```python
from build123d import *

# Parameters (mm, degrees)
F1_DEPTH = 1
F3_DEPTH = 2
F4_W     = 19.942
F4_H     = 20.917
F5_DEPTH = 2
F2_W     = 2.335
F2_H     = 6.803
F6_DEPTH = 6
F7_W     = 10.966
F7_H     = 10.966
F8_DEPTH = 1


with BuildPart() as f1:
    # F0 (on Top) → F1 (new body)
    with BuildSketch(Plane.XY):
        with BuildLine():
            Line((-9.672, -16.5), (8.5, -16.5))
            ThreePointArc((8.5, -16.5), (14.156854, -14.156854), (16.5, -8.5))
            Line((16.5, -8.5), (16.5, 8.5))
            ThreePointArc((16.5, 8.5), (14.156854, 14.156854), (8.5, 16.5))
            Line((8.5, 16.5), (-9.672, 16.5))
            ThreePointArc((-9.672, 16.5), (-14.500125, 14.500125), (-16.5, 9.672))
            Line((-16.5, 9.672), (-16.5, -9.672))
            ThreePointArc((-16.5, -9.672), (-14.500125, -14.500125), (-9.672, -16.5))
        make_face()
    extrude(amount=F1_DEPTH)

    # F2 (on face) → F3 (join)
    with BuildSketch(Plane.XY.offset(1)):
        with BuildLine():
            Line((16.317289, -10.2), (17.5, -10.2))
            Line((17.5, -10.2), (17.5, -0.2))
            Line((17.5, -0.2), (16.5, -0.2))
            Line((16.5, -0.2), (16.5, -8.5))
            ThreePointArc((16.5, -8.5), (16.454191, -9.354895), (16.317289, -10.2))
        make_face()
        with BuildLine():
            Line((10.5, -10.2), (16.317289, -10.2))
            ThreePointArc((16.317289, -10.2), (16.454191, -9.354895), (16.5, -8.5))
            Line((16.5, -8.5), (16.5, -0.2))
            Line((16.5, -0.2), (10.5, -0.2))
            Line((10.5, -0.2), (10.5, -10.2))
        make_face()
    extrude(amount=F3_DEPTH)

    # F4 (on face) → F5 (join)
    with BuildSketch(Plane.XY.offset(1)):
        Rectangle(F4_W, F4_H)
    extrude(amount=F5_DEPTH)

    # F2 (on face) → F6 (join)
    with BuildSketch(Plane.XY.offset(1)):
        with Locations((14.3325, 5.7395)):
            Rectangle(F2_W, F2_H)
    extrude(amount=F6_DEPTH)

    # F7 (on face) → F8 (join)
    with BuildSketch(Plane(origin=(0, 0, 0), x_dir=(1, 0, 0), z_dir=(0, 0, -1))):
        with Locations((-6.651, 0.863)):
            Rectangle(F7_W, F7_H)
    extrude(amount=F8_DEPTH)


solid = f1.part
```
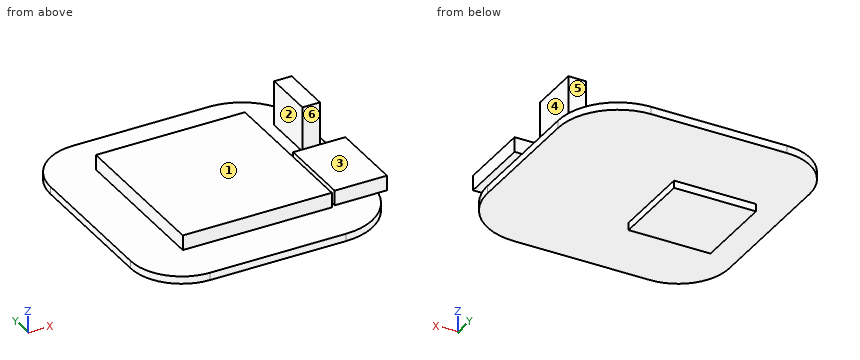
Verification items for the finished model (mm, model axes). Face numbers are marked on the shaded views. A direction names the side the tool comes from. Give positions to 0.01 mm unless a question says otherwise; leave off trailing zeros. Order: outer loops, then holes, each group sorted by start corner. A loop starts at its lowest first (then second) coordinate and runs counter-clockwise, first axis right, second up. Notation, with made-up numbers: M 14.25,-4.5 L 41.25,-4.5 A17 cw 41.25,20.5 Z; hole C 41,85.25 d5. An arc over 180 degrees is marked long. Return JSON: item names as keys, results as strings. Group by question number.
1) Go/stop test with flat-tipped pins: pin 1 Ø1.2 at (x, z) = (14, 5.5) entering from -Y; pin 2 Ø2 at (x, z) = (12.5, 2.5) entering from -Y; pin 3 Ø7.5 at (x, y) = (15, -6.5) entering from +Z. Record where each tip stops, or that it passes through.
2) Scan lines: line 1 (Z direction, x = -13.5, y = -11); line 2 (Z direction, x = -8, y = 4); line 3 (X direction, y = -4, z = 0.25). Record each from-to range of solid material in increasing order.
3) Section check B-B on z = 2.25. Record the cut outline in (x, y) (1 decimal), and give its area (3 significant figures).
4) Mould release check, pull along Y, two halves, no side actions. Record for the marked faces 4, 5 and 6: pulls with the +Y half, pulls with the -Y half, needs draft (parallel to the pull), parting line crosses it, or undercut.
5) Access from +Z, -Z, +X, -X, +Y, -Y to the whole of each face (thin tool, end or side, straight path). Record for the marked faces 1, 2 and 3.
6) Section check C-C on y = 8. Record the cut outline in (x, z) (3 decimals).
7) Section check A-A on x = -4.5. Record the cut outline in (y, z), and give its area (3 significant figures).
8) Section check D-D on z = 4.75. Record the cut outline in (x, y) (3 decimals).
Answer block:
{
 "1": {"pin 1": "stops at y = 2.34", "pin 2": "stops at y = -10.2", "pin 3": "stops at z = 3"},
 "2": {"line 1": "z = 0 to 1", "line 2": "z = -1 to 3", "line 3": "x = -16.5 to 16.5"},
 "3": {"outline": "M -10,-10.5 L 10,-10.5 L 10,10.5 L -10,10.5 Z; M 10.5,-10.2 L 17.5,-10.2 L 17.5,-0.2 L 10.5,-0.2 Z; M 13.2,2.3 L 15.5,2.3 L 15.5,9.1 L 13.2,9.1 Z", "area": "503 mm^2"},
 "4": {"face 4": "needs draft", "face 5": "pulls with the +Y half", "face 6": "undercut"},
 "5": {"face 1": "+Z, -X, +Y, -Y", "face 2": "+Z, +Y", "face 3": "+Z, +X, -X, -Y"},
 "6": {"outline": "M -16.5,0 L 16.5,0 L 16.5,1 L 15.5,1 L 15.5,7 L 13.165,7 L 13.165,1 L 9.971,1 L 9.971,3 L -9.971,3 L -9.971,1 L -16.5,1 Z"},
 "7": {"outline": "M -16.5,0 L -6.35,0 L -6.35,-1 L 4.62,-1 L 4.62,0 L 16.5,0 L 16.5,1 L 10.46,1 L 10.46,3 L -10.46,3 L -10.46,1 L -16.5,1 Z", "area": "85.8 mm^2"},
 "8": {"outline": "M 13.165,2.338 L 15.5,2.338 L 15.5,9.141 L 13.165,9.141 Z"}
}
